Autodesk Inventor part; units mm, degrees
ref_plane "YZ Plane" through (0, 0, 0) normal (1, 0, 0) x (0, 1, 0)
ref_plane "XZ Plane" through (0, 0, 0) normal (0, 1, 0) x (-1, 0, 0)
ref_plane "XY Plane" through (0, 0, 0) normal (0, 0, 1) x (1, 0, 0)
sketch "Sketch1" plane through (0, 0, 0) normal (0, 1, 0) x (-1, 0, 0)
  line L0 (0, 0) -> (8, 0)
  line L1 (8, 0) -> (8, -80)
  line L2 (0, -80) -> (0, 0)
  line L3 (8, -80) -> (57.5929, -216.2554)
  line L4 (8, -80) -> (153, -80) construction
  line L5 (57.5929, -216.2554) -> (50.0754, -218.9916)
  line L6 (50.0754, -218.9916) -> (0.4825, -82.7362)
  line L7 (0.4825, -82.7362) -> (0, -81.4106)
  line L8 (0, -81.4106) -> (0, -80)
  dimension "d3" = 8
  dimension "d4" = 80
  dimension "d6" = 70
  dimension "d7" = 8
extrude "Extrusion1" add sketch "Sketch1" along normal blind 8
sketch "Sketch2" plane through (-8, 0, 0) normal (0, 0, 1) x (1, 0, 0)
  line L0 (8, 8) -> (8, 15)
  line L1 (8, 8) -> (0, 8)
  line L2 (8, 8) -> (-42.0754, 8)
  line L3 (0, 8) -> (0, 15)
  line L4 (0, 15) -> (8, 15)
  point P0 (8, 0)
  dimension "d10" = 7
  dimension "d11" = 8
extrude "Extrusion2" add sketch "Sketch2" against normal blind 80
sketch "Sketch3" plane through (-57.5929, 0, -216.2554) normal (-0.342, 0, -0.9397) x (-0.9397, 0, 0.342)
  line L0 (-8, 0) -> (-8, 8)
  line L1 (0, 0) -> (0, 8)
  line L2 (-8, 8) -> (0, 8)
  line L3 (-7.5175, 15) -> (-7.5175, 8)
  line L4 (-8, 8) -> (-8, 15)
  line L5 (0, 8) -> (0, 15)
  line L6 (0, 15) -> (-8, 15)
  point P0 (19.8441, 0)
  dimension "d14" = 8
extrude "Extrusion3" add sketch "Sketch3" against normal blind 145
sketch "Sketch8" plane through (0, 0, 0) normal (0, -1, 0) x (1, 0, 0)
  line L0 (-8, -80) -> (-8, 0)
  line L1 (-8, -80) -> (0, -80)
  line L2 (0, -80) -> (0, -104)
  line L3 (0, -104) -> (-8, -104)
  line L4 (-8, -104) -> (-8, -80)
  circle A0 centre (-4, -100) radius 2.2
  circle A1 centre (-4, -84) radius 2.2
  point P0 (0, 0)
  point P1 (-4, -80)
  point P2 (-4, -104)
  dimension "d24" = 24
  dimension "d25" = 4.4
  dimension "d26" = 4.4
  dimension "d27" = 4
  dimension "d28" = 4
extrude "Extrusion7" add sketch "Sketch8" against normal blind 15
sketch "Sketch9" plane through (0, 15, 0) normal (0, 1, 0) x (1, 0, 0)
  line L0 (0, 80) -> (0, 104)
  line L1 (-8, 80) -> (-0.4825, 82.7362)
  line L2 (0, 104) -> (-8, 104)
  line L3 (-8, 104) -> (-8, 80)
  line L4 (-8, 80) -> (0, 80)
  line L5 (0, 80) -> (0, 104)
  point P0 (0, 0)
extrude "Extrusion8" cut sketch "Sketch9" along normal blind 145
extrude "Extrusion9" cut sketch "Sketch8" against normal blind 24 contours A1
sketch "Sketch10" plane through (0, 0, 0) normal (0, -1, 0) x (1, 0, 0)
  line L0 (0, -104) -> (-8, -104)
  line L1 (0, 0) -> (0, -104)
  line L2 (-8, -104) -> (0, -104)
  line L3 (0, -104) -> (0, -80)
  line L4 (0, -80) -> (-8, -80)
  line L5 (-8, -80) -> (-8, -104)
  dimension "d47" = 24
extrude "Extrusion10" cut sketch "Sketch10" against normal blind 5
sketch "Sketch11" plane through (0, 5, 0) normal (0, -1, 0) x (1, 0, 0)
  line L0 (0, -104) -> (-8, -104)
  line L1 (-50.0754, -218.9916) -> (-8, -103.3904)
  line L2 (0, -104) -> (-8, -104)
  line L3 (-8, -104) -> (-8, -103.3904)
  line L4 (-8, -103.3904) -> (0, -103.3904)
  line L5 (0, -103.3904) -> (0, -104)
  point P0 (0, 0)
extrude "Extrusion11" cut sketch "Sketch11" against normal blind 13
chamfer "Chamfer3" distance 7 angle 84 1 edges at (-4, 0, 0) measured on face at (-5.3333, 5, 0)
chamfer "Chamfer4" distance 7 angle 75 1 edges at (-53.8342, 0, -217.6235) measured on face at (-55.0871, 5, -217.1675)
properties part number "intake arm right"
Source: CAD feature listing. Evaluate the final solid. Frame: model axes, mm. A direction names the side the tool comes from. Coordinates: 2 decimals unless noted, no trailing zeros. Loops run counter-clockwise (first coordinate to the right, second up) from the corner with the lowest first, then second, coordinate; pieces in that order, holes last. Notation, with made-up numbers: (-17.75, 39) -> (-0.75, 39) arc R10 ccw to (-0.75, 50) -> close; hole circle Ø5 at (85, -24.75). An arc over 180 degrees is marked (long way). Answer in a Markdown table with one row per item. Add a question column.
Q1. Section B-B on x = -4. Return the cut outline in (y, z), and give its area (3 significant figures).
Q2. Reachability of faces 5 (the face through (-4, 5, -92)), 6 (the face through (-4, 10, -103.39)), 7 (the face through (-49.25, 3.45, -205.2)) from +Z, -Z, +X, -X, +Y, -Y: full face, straight path, thin tool, end or side. Return the list, or none.
Q3. Ray query, line 1 along Z through (x, y) = (-4, 8); line 2 along Y through (x, z) = (-4.5, -86.5); line 3 along X through (y, z) = (8.25, -29.5). Return the intervals inside material, ascending.
Q4. Section A-A on y = 11. Give the number of separate pieces and of enclosed holes in the cut face, and give its area (3 significant figures).
Q5. Section C-C on z = -100. Return the cut outline in (x, y), and give its area (3 significant figures).
Q6. Pull-direction query (Z, two-part tool) for faces 1 (the face through (-2.817, 9.93, -82.145)), 2 (the face through (-2.817, 9.93, -98.145)), 3 (the face through (-53.782, 11.549, -217.643)), 4 (the face through (-8, 9, -39)); classes: pulls with the +Z half, pulls with the -Z half, needs draft (parallel to the pull), parting line crosses it, or undercut.
Q7. Contact query for flat-ended pins moving along their axis: pin 1 Ø4.5 at (y, z) = (4, -50.5) entering from -X; pin 2 Ø4 at (x, z) = (-5.5, -91) entering from -Y; pin 3 Ø2.5 at (x, y) = (-2.5, 10.5) entering from -Z. Output: stop coordinate, or through.
Computed values:
| question | item | result |
|---|---|---|
| 1 | outline | (0, -80) -> (5, -80) -> (5, -81.8) -> (15, -81.8) -> (15, 0) -> (7, 0) -> (0, -66.6) -> close; (5, -103.39) -> (15, -103.39) -> (15, -102.2) -> (5, -102.2) -> close; (5, -97.8) -> (15, -97.8) -> (15, -86.2) -> (5, -86.2) -> close |
| 1 | area | 1,110 mm^2 |
| 2 | face 5 | -Z, +X, -Y |
| 2 | face 6 | -Z, +X, +Y, -Y |
| 2 | face 7 | -Z, -X, -Y |
| 3 | line 1 | z = -103.39 to -102.2, -97.8 to -86.2, -81.8 to 0 |
| 3 | line 2 | y = 5 to 15 |
| 3 | line 3 | x = -8 to 0 |
| 4 | separate pieces | 1 |
| 4 | enclosed holes | 2 |
| 4 | area | 1,870 mm^2 |
| 5 | outline | (-15.28, 0) -> (-8, 0) -> (-8, 5) -> (-6.2, 5) -> (-6.2, 15) -> (-15.28, 15) -> close; (-1.8, 5) -> (0, 5) -> (0, 15) -> (-1.8, 15) -> close |
| 5 | area | 145 mm^2 |
| 6 | face 1 | undercut |
| 6 | face 2 | undercut |
| 6 | face 3 | pulls with the -Z half |
| 6 | face 4 | needs draft |
| 7 | pin 1 | stops at x = -8 |
| 7 | pin 2 | stops at y = 5 |
| 7 | pin 3 | stops at z = -103.39 |
